```python
from build123d import *

# Parameters (mm, degrees)
EXTRUDE_1_DEPTH = 5


with BuildPart() as part:
    # 草圖1 → 填料-伸長1 (new body)
    with BuildSketch(Plane(origin=(0, 0, 0), x_dir=(1, 0, 0), z_dir=(0, 1, 0))):
        Polygon((-29.65648855, 0), (-29.65648855, 32.5), (-13.65648855, 32.5), (-13.65648855, 2.1), (40.34351145, 2.1), (40.34351145, 0), (-16.60648855, 0), (-16.60648855, 27.5), (-26.70648855, 27.5), (-26.70648855, 0), align=None)
    extrude_1 = extrude(amount=EXTRUDE_1_DEPTH)

    # 鏡射1: 填料-伸長1 across plane
    add(extrude_1.mirror(Plane(origin=(-16.60648855, 5, 0), x_dir=(1, 0, 0), z_dir=(0, 0, -1))))


solid = part.part
```
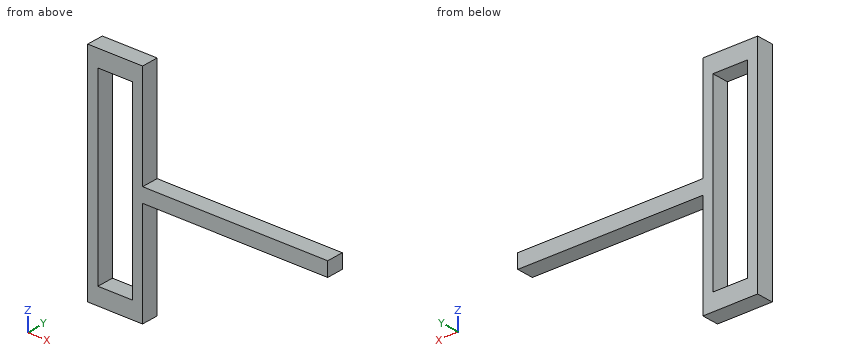
Design review of the part built by this model. Coordinates are the model's own, in mm. Coordinates: 2 decimals unless noted, no trailing zeros. Order: outer loops, then holes, each group sorted by start corner. A loop starts at its lowest first (then second) coordinate and runs counter-clockwise, first axis right, second up.
1) Take a section at D-D, the plane x = -9.5. Give the boundary of the cut face in (y, z), and give its area (3 significant figures).
2) Wall thickness on line 1 along Z through (x, y) = (-21, 0.4); line 2 along X through (y, z) = (3.6, -26); line 3 along Z through (x, y) = (-4.5, 3.95): over which ranges is each line inside the solid? List them lowest first.
3) Take a section at B-B, the plane x = -17.5. Give the boundary of the cut face in (y, z).
4) Clearance check with flat-ended pins moving along their axes: pin 1 (1.5 mm diameter, centred on x = -12, z = 7, fed in from -Y); pin 2 (1.5 mm diameter, centred on y = 3, z = -13.5, fed in from +X); pin 3 (2.5 mm diameter, centred on x = 8.5, y = 3, fed in from +Z). State where each tip first meets the part, or that it passes through.
5) Take a section at A-A, the plane z = 20.5. Give the boundary of the cut face in (x, y).
6) Take a section at C-C, the plane y = 4.1. Give the boundary of the cut face in (x, z), and give its area (3 significant figures).
Returned:
1. outline: (0, -2.1) - (5, -2.1) - (5, 2.1) - (0, 2.1) - close
1. area: 21.0 mm2
2. line 1: z = -32.5 to -27.5, 27.5 to 32.5
2. line 2: x = -29.66 to -26.71, -16.61 to -13.66
2. line 3: z = -2.1 to 2.1
3. outline: (0, -32.5) - (5, -32.5) - (5, -27.5) - (0, -27.5) - close; (0, 27.5) - (5, 27.5) - (5, 32.5) - (0, 32.5) - close
4. pin 1: passes through
4. pin 2: stops at x = -13.66
4. pin 3: stops at z = 2.1
5. outline: (-29.66, 0) - (-26.71, 0) - (-26.71, 5) - (-29.66, 5) - close; (-16.61, 0) - (-13.66, 0) - (-13.66, 5) - (-16.61, 5) - close
6. outline: (-29.66, -32.5) - (-13.66, -32.5) - (-13.66, -2.1) - (40.34, -2.1) - (40.34, 2.1) - (-13.66, 2.1) - (-13.66, 32.5) - (-29.66, 32.5) - close; hole (-26.71, -27.5) - (-16.61, -27.5) - (-16.61, 27.5) - (-26.71, 27.5) - close
6. area: 711 mm2
